```python
from build123d import *

# Parameters (mm, degrees)
SKETCH4_W           = 31.1
SKETCH4_H           = 19.1
BOSS_EXTRUDE1_DEPTH = 19
SHELL1_T            = 2
SKETCH5_W           = 12
SKETCH5_H           = 19.1
CUT_EXTRUDE1_DEPTH  = 2


with BuildPart() as part:
    # Sketch4 → Boss-Extrude1 (new body)
    with BuildSketch(Plane(origin=(0, 0, 0), x_dir=(0, 0, -1), z_dir=(1, 0, 0))):
        Rectangle(SKETCH4_W, SKETCH4_H)
    extrude(amount=BOSS_EXTRUDE1_DEPTH)

    # Shell1
    shell1_openings = [part.faces().sort_by_distance(p)[0] for p in [
        (0, 0, 0),
    ]]
    offset(amount=SHELL1_T, openings=shell1_openings, kind=Kind.INTERSECTION)

    # Sketch5 → Cut-Extrude1 (cut)
    with BuildSketch(Plane(origin=(0, 0, -17.55), x_dir=(-1, 0, 0), z_dir=(0, 0, -1))):
        with Locations((-6, 0)):
            Rectangle(SKETCH5_W, SKETCH5_H)
    extrude(amount=-CUT_EXTRUDE1_DEPTH, mode=Mode.SUBTRACT)


solid = part.part
```
Geometry: final body of the model. Coordinates: model frame, mm. A direction names the side the tool comes from. Coordinates: 2 decimals unless noted, no trailing zeros. Write each loop counter-clockwise with the first axis right and the second up, starting at its lowest first coordinate (ties: lowest second). Pieces come first, ordered by that corner, then holes. Notation, with made-up numbers: M -37,2.25 L 21,2.25 A27 cw 21,23.25 Z; hole C -26,65 d4. An arc over 180 degrees is marked long. Use CSV: the item, a comma, the result in double quotes. Start each with the question number.
1. Mould query, pull axis Y, two halves, no side actions, for faces 1 (the face through (10, 11.55, 0)), 2 (the face through (12, 0, -17)), 3 (the face through (9, 9.55, -1)), 4 (the face through (10, -11.55, 0)). Classes: pulls with the +Y half, pulls with the -Y half, needs draft (parallel to the pull), parting line crosses it, or undercut.
2. Ray query, probe 1 along Z at (x, y) = (14.75, -6.25); probe 2 along Y at (x, z) = (5.5, -5); probe 3 along Z at (x, y) = (1.5, -3.25). Return the intervals inside material, ascending.
3. First-contact query: P1, Ø2, axis at y = 1, z = 13, coming from the -X side; P2, Ø1.6, axis at y = 0, z = -16.5, coming from the -X side; P3, Ø10, axis at x = 9.5, y = 3.5, coming from the -Z side. Flat tips, straight axial feed; report the tip coordinate or a pass-through.
4. Cut plane A-A on x = 14.25. Return the cut outline in (y, z).
5. Cut plane B-B on z = -1. Return the cut outline in (x, y), plus the area to 3 significant figures.
6. Cut plane C-C on y = 0.25. Return the cut outline in (x, z), plus the area to 3 significant figures.
7. Reachability of faces 5 (the face through (10, 0, 17.55)), 6 (the face through (9, -9.55, -1)) from +Z, -Z, +X, -X, +Y, -Y: full face, straight path, thin tool, end or side. Return the list, or none.
Entries:
1,face 1,"pulls with the +Y half"
1,face 2,"undercut"
1,face 3,"undercut"
1,face 4,"pulls with the -Y half"
2,probe 1,"-17.55 to -15.55, 15.55 to 17.55"
2,probe 2,"-11.55 to -9.55, 9.55 to 11.55"
2,probe 3,"15.55 to 17.55"
3,P1,"x = 19"
3,P2,"x = 12"
3,P3,"z = -17.55"
4,outline,"M -11.55,-17.55 L 11.55,-17.55 L 11.55,17.55 L -11.55,17.55 Z; hole M -9.55,-15.55 L 9.55,-15.55 L 9.55,15.55 L -9.55,15.55 Z"
5,outline,"M 0,-11.55 L 21,-11.55 L 21,11.55 L 0,11.55 L 0,9.55 L 19,9.55 L 19,-9.55 L 0,-9.55 Z"
5,area,"122 mm²"
6,outline,"M 0,15.55 L 19,15.55 L 19,-15.55 L 12,-15.55 L 12,-17.55 L 21,-17.55 L 21,17.55 L 0,17.55 Z"
6,area,"122 mm²"
7,face 5,"+Z, +X, -X, +Y, -Y"
7,face 6,"-X"
